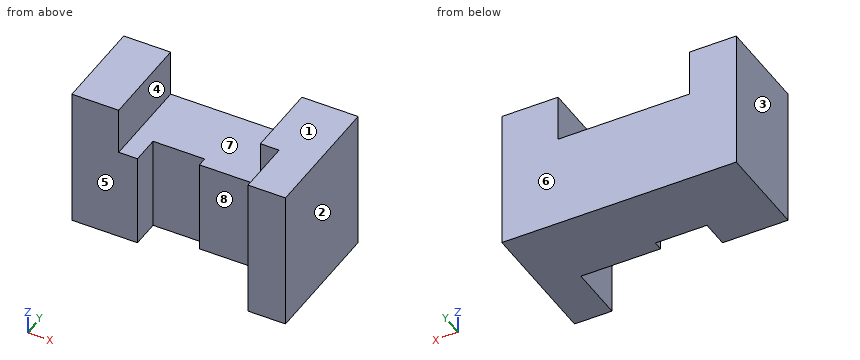
```python
from build123d import *

# Parameters (mm, degrees)
F0_W     = 70
F0_H     = 75
F1_DEPTH = 62.5
F3_DEPTH = 75.001
F4_W     = 70
F4_H     = 25
F5_DEPTH = 70.001


with BuildPart() as f1:
    # F0 (on Right) → F1 (new body, symmetric)
    with BuildSketch(Plane.YZ):
        with Locations((0, 37.5)):
            Rectangle(F0_W, F0_H)
    extrude(amount=F1_DEPTH, both=True)

    # F2 (on face) → F3 (cut, through all)
    with BuildSketch(Plane.XY.offset(75)):
        Polygon((-62.5, -15), (-62.5, -35), (42.5, -35), (42.5, -5), (0, -5), (0, 0), (-27.5, 0), (-27.5, -15), align=None)
    extrude(amount=-F3_DEPTH, mode=Mode.SUBTRACT)

    # F4 (on face) → F5 (cut, through all)
    with BuildSketch(Plane(origin=(0, 35, 0), x_dir=(-1, 0, 0), z_dir=(0, 1, 0))):
        with Locations((2.5, 62.5)):
            Rectangle(F4_W, F4_H)
    extrude(amount=-F5_DEPTH, mode=Mode.SUBTRACT)


solid = f1.part
```
Geometry: final body of the model. Coordinates: model frame, mm. Face numbers are marked on the shaded views. A direction names the side the tool comes from. Coordinates: 2 decimals unless noted, no trailing zeros. Loops run counter-clockwise (first coordinate to the right, second up) from the corner with the lowest first, then second, coordinate; pieces in that order, holes last. Notation, with made-up numbers: M -31.5,21 L 23.5,21 A18 ccw 23.5,40 Z; hole C -25.75,60 d8. An arc over 180 degrees is marked long. Put each result on its own line as item: value.
(1) Draft query along X for the marked faces 1, 2, 3 and 4. Return one class per face: pulls with the +X half, pulls with the -X half, needs draft (parallel to the pull), parting line crosses it, or undercut.
Answer sheet:
face 1: needs draft
face 2: pulls with the +X half
face 3: pulls with the -X half
face 4: undercut
(2) Cut plane B-B on z = 45. Return the cut outline in (x, y).
Answer sheet:
outline: M -62.5,-15 L -27.5,-15 L -27.5,0 L 0,0 L 0,-5 L 42.5,-5 L 42.5,-35 L 62.5,-35 L 62.5,35 L -62.5,35 Z
(3) First-contact query: pin 1 (10.5 mm diameter, centred on x = -40.5, z = 47.5, fed in from -Y); pin 2 (15 mm diameter, centred on y = -24, z = 42, fed in from -X); pin 3 (1 mm diameter, centred on x = 5, y = -3, fed in from +Z). Flat tips, straight axial feed; report the tip coordinate or a pass-through.
Answer sheet:
pin 1: stops at y = -15
pin 2: stops at x = 42.5
pin 3: stops at z = 50
(4) Cut plane D-D on x = 36.5. Return the cut outline in (y, z), then the cut area to 3 significant figures.
Answer sheet:
outline: M -5,0 L 35,0 L 35,75 L -5,75 Z
area: 3,000 mm^2
(5) Access query for the marked faces 5, 6, 7 and 8. Directions: +Z, -Z, +X, -X, +Y, -Y. A direction counts if a zero-diameter tool reaches every point of the face in a straight line with its end or side. Return the directions, or none.
Answer sheet:
face 5: +Z, -Z, -X, -Y
face 6: +Z, -Z, +X, -X, +Y
face 7: +Z, +Y, -Y
face 8: +Z, -Z, -Y
(6) Material intervals for probe 1 along X at (y, z) = (-1, 44.5); probe 2 along X at (y, z) = (-10, 61.5); probe 3 along X at (y, z) = (-29, 15), sorted ascending.
Answer sheet:
probe 1: x = -62.5 to -27.5, 0 to 62.5
probe 2: x = -62.5 to -37.5, 42.5 to 62.5
probe 3: x = 42.5 to 62.5
(7) Cut plane A-A on y = 20. Return the cut outline in (x, z).
Answer sheet:
outline: M -62.5,0 L 62.5,0 L 62.5,75 L 32.5,75 L 32.5,50 L -37.5,50 L -37.5,75 L -62.5,75 Z
(8) Cut plane C-C on z = 70. Return the cut outline in (x, y), then the cut area to 3 significant figures.
Answer sheet:
outline: M -62.5,-15 L -37.5,-15 L -37.5,35 L -62.5,35 Z; M 32.5,-5 L 42.5,-5 L 42.5,-35 L 62.5,-35 L 62.5,35 L 32.5,35 Z
area: 3,050 mm^2
